Source: CAD feature listing. Evaluate the final solid. Frame: model axes, mm. Face numbers are marked on the shaded views. A direction names the side the tool comes from. Round coordinates to 2 decimals unless told otherwise and drop trailing zeros. Write each loop counter-clockwise with the first axis right and the second up, starting at its lowest first coordinate (ties: lowest second). Pieces come first, ordered by that corner, then holes.
from build123d import *

# Parameters (mm, degrees)
F0_W     = 76.2
F0_H     = 76.2
F1_DEPTH = 7.62
F3_DEPTH = 12.7
F4_R     = 4.137454
F5_DEPTH = 25.4


with BuildPart() as f1:
    # F0 (on Top) → F1 (new body)
    with BuildSketch(Plane.XY):
        Rectangle(F0_W, F0_H)
    extrude(amount=F1_DEPTH)

    # F2 (on face) → F3 (join)
    with BuildSketch(Plane.XY.offset(7.62)):
        Polygon((-20.543544, 0), (0, -20.543544), (20.543544, 0), (0, 20.543544), align=None)
    extrude(amount=F3_DEPTH)

    # F4 (on face) → F5 (join)
    with BuildSketch(Plane(origin=(0, 0, 0), x_dir=(1, 0, 0), z_dir=(0, 0, -1))):
        Circle(F4_R)
    extrude(amount=F5_DEPTH)


solid = f1.part
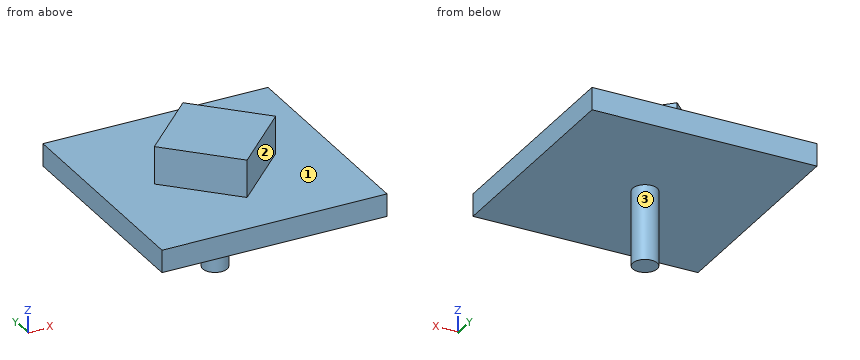
1) Section query D-D on y = 16.5. Return the cut outline in (x, z).
Taken from the geometry:
outline: (-38.1, 0) - (38.1, 0) - (38.1, 7.62) - (4.04, 7.62) - (4.04, 20.32) - (-4.04, 20.32) - (-4.04, 7.62) - (-38.1, 7.62) - close
2) Contact query for flat-ended pins moving along their axis: P1, Ø5, axis at y = 6.5, z = 10.5, coming from the -X side; P2, Ø1, axis at x = -19.5, y = -18.5, coming from the +Z side; P3, Ø10, axis at y = 23, z = 15.5, coming from the +X side; P4, Ø4, axis at x = -8, z = -11.5, coming from the -Y side. Output: stop coordinate, or through.
Taken from the geometry:
P1: stops at x = -16.54
P2: stops at z = 7.62
P3: stops at x = 2.54
P4: passes through
3) Section query A-A on y = 2.5. Return the cut outline in (x, z), then the cut area to 3 significant figures.
Taken from the geometry:
outline: (-38.1, 0) - (-3.3, 0) - (-3.3, -25.4) - (3.3, -25.4) - (3.3, 0) - (38.1, 0) - (38.1, 7.62) - (18.04, 7.62) - (18.04, 20.32) - (-18.04, 20.32) - (-18.04, 7.62) - (-38.1, 7.62) - close
area: 1,210 mm2
4) Section query B-B on x = -10. Return the cut outline in (y, z), then the cut area to 3 significant figures.
Taken from the geometry:
outline: (-38.1, 0) - (38.1, 0) - (38.1, 7.62) - (10.54, 7.62) - (10.54, 20.32) - (-10.54, 20.32) - (-10.54, 7.62) - (-38.1, 7.62) - close
area: 848 mm2
5) Material intervals for line 1 (Z direction, x = -3, y = -7); line 2 (Z direction, x = -11.5, y = 14.5); line 3 (Y direction, x = -4, z = 11.5), sorted ascending.
Taken from the geometry:
line 1: z = 0 to 20.32
line 2: z = 0 to 7.62
line 3: y = -16.54 to 16.54
6) Section query C-C on z = 14.5. Return the cut outline in (x, y).
Taken from the geometry:
outline: (-20.54, 0) - (0, -20.54) - (20.54, 0) - (0, 20.54) - close
7) Reachability of the marked faces 1, 2 and 3 from +Z, -Z, +X, -X, +Y, -Y: full face, straight path, thin tool, end or side. Return the list, or none.
Taken from the geometry:
face 1: +Z
face 2: +Z, +X, -Y
face 3: -Z
